Could you check a few things on this model? Use its own coordinates, in mm. A direction names the side the tool comes from. Round coordinates to 2 decimals unless told otherwise and drop trailing zeros. Loops run counter-clockwise (first coordinate to the right, second up) from the corner with the lowest first, then second, coordinate; pieces in that order, holes last. Notation, with made-up numbers: (-18.5, 39) -> (-2.5, 39) arc R11 cw to (-2.5, 53) -> close; hole circle Ø10 at (71.25, 40.25). An arc over 180 degrees is marked (long way). One line per item, written item: value.
```python
from build123d import *

# Parameters (mm, degrees)
F1_DEPTH = 20
F2_R     = 5
F4_R     = 2.5
F5_DEPTH = 62.5836819879


with BuildPart() as f1:
    # F0 (on Front) → F1 (new body, symmetric)
    with BuildSketch(Plane.XZ):
        with BuildLine():
            Line((37.7684786426, 214.1956862802), (38.6367195309, 219.1197250452))
            ThreePointArc((38.6367195309, 219.1197250452), (0, 222.5), (-38.6367195309, 219.1197250452))
            Line((-38.6367195309, 219.1197250452), (-37.7684786426, 214.1956862802))
            ThreePointArc((-37.7684786426, 214.1956862802), (-2.5001651855, 217.4856298104), (32.8344587783, 215.0073215422))
            ThreePointArc((32.8344587783, 215.0073215422), (35.3038012268, 214.6156835344), (37.7684786426, 214.1956862802))
        make_face()
        with BuildLine():
            Line((30.3884310917, 172.3413567771), (37.7684786426, 214.1956862802))
            ThreePointArc((37.7684786426, 214.1956862802), (35.3038012268, 214.6156835344), (32.8344587783, 215.0073215422))
            Line((32.8344587783, 215.0073215422), (25.451986353, 173.1392398929))
            ThreePointArc((25.451986353, 173.1392398929), (27.9230587413, 172.7579311943), (30.3884310917, 172.3413567771))
        make_face()
        with BuildLine():
            Line((29.5201902034, 167.4173180121), (30.3884310917, 172.3413567771))
            ThreePointArc((30.3884310917, 172.3413567771), (27.9230587413, 172.7579311943), (25.451986353, 173.1392398929))
            ThreePointArc((25.451986353, 173.1392398929), (-2.5002551932, 174.9821382998), (-30.3884310917, 172.3413567771))
            Line((-30.3884310917, 172.3413567771), (-29.5201902034, 167.4173180121))
            ThreePointArc((-29.5201902034, 167.4173180121), (0, 170), (29.5201902034, 167.4173180121))
        make_face()
    extrude(amount=F1_DEPTH, both=True)

    # F2
    f2_edges = [f1.edges().sort_by_distance(p)[0] for p in [
        (38.63672, 0, 219.119725),
        (32.834459, 0, 215.007322),
        (29.52019, 0, 167.417318),
        (25.451986, 0, 173.13924),
    ]]
    fillet(f2_edges, radius=F2_R)

    # F4 (on offset) → F5 (cut, through all)
    with BuildSketch(Plane.XY.offset(230)):
        with Locations((0, 12.5)):
            Circle(F4_R)
        with Locations((0, -12.5)):
            Circle(F4_R)
    extrude(amount=-F5_DEPTH, mode=Mode.SUBTRACT)


solid = f1.part
```
(1) Imagine slicing it at A-A on x = 0. Write out the boundary of the cut face in (y, z).
Results below:
outline: (-20, 170) -> (-15, 170) -> (-15, 175) -> (-20, 175) -> close; (-20, 217.5) -> (-15, 217.5) -> (-15, 222.5) -> (-20, 222.5) -> close; (-10, 170) -> (10, 170) -> (10, 175) -> (-10, 175) -> close; (-10, 217.5) -> (10, 217.5) -> (10, 222.5) -> (-10, 222.5) -> close; (15, 170) -> (20, 170) -> (20, 175) -> (15, 175) -> close; (15, 217.5) -> (20, 217.5) -> (20, 222.5) -> (15, 222.5) -> close
(2) Imagine slicing it at B-B on x = -15. Write out the boundary of the cut face in (y, z), then the cut area to 3 significant figures.
Results below:
outline: (-20, 169.34) -> (20, 169.34) -> (20, 174.36) -> (-20, 174.36) -> close; (-20, 216.98) -> (20, 216.98) -> (20, 221.99) -> (-20, 221.99) -> close
area: 401 mm²
(3) Imagine slicing it at D-D on y = 12.5. Give the number of separate pieces and of enclosed holes in the cut face, then the cut area to 3 significant figures.
Results below:
separate pieces: 3
enclosed holes: 0
area: 848 mm²
(4) Please list where these lines run through material, in increasing order: L1, parallel to Y at x = 0, z = 173; L2, parallel to Z at x = 0, y = 0; L3, parallel to Z at x = 4.5, y = 8.
Results below:
L1: y = -20 to -15, -10 to 10, 15 to 20
L2: z = 170 to 175, 217.5 to 222.5
L3: z = 169.94 to 174.94, 217.45 to 222.45
(5) On a 3-axis mill with a long thin cutter (end or side, diameter ignored), from which of +Z, -Z, +X, -X, +Y, -Y can I reach the whole of each face in a straight line? I mean faces 4 (the face through (5, 20, 218)), 5 (the face through (24.298, -0.28, 174.682)), 6 (the face through (29.15, -0.28, 194.11)). Say none if no direction works.
Results below:
face 4: +Z, -Z, +X, -X, +Y
face 5: +Y, -Y
face 6: -X, +Y, -Y
(6) We'd pull the mould along Z, two halves only. Please class faces 1 (the face through (-0.54, 10.06, 220.03)), 2 (the face through (-29.96, -0.28, 169.91)), 3 (the face through (-4.504, -0.28, 174.942)): +Z half, -Z half, draft (parallel to the pull), parting line (faces both ways), or undercut.
Results below:
face 1: draft
face 2: -Z half
face 3: undercut
(7) Imagine slicing it at C-C on x = -24.5. Write out the boundary of the cut face in (y, z), then the cut area to 3 significant figures.
Results below:
outline: (-20, 168.23) -> (20, 168.23) -> (20, 173.28) -> (-20, 173.28) -> close; (-20, 216.12) -> (20, 216.12) -> (20, 221.15) -> (-20, 221.15) -> close
area: 403 mm²
(8) For pin 1 Ø6 at (y, z) = (0, 195.5) entering from +X; pin 2 Ø6.5 at (x, y) = (0, -12.5) entering from -Z; pin 3 Ø5 at (y, z) = (14.5, 195) entering from -X; pin 4 Ø4 at (x, y) = (0, 12.5) entering from +Z, each with a flat end and sliding along its axis, tell me the tip position at first contact or that it passes through.
Results below:
pin 1: stops at x = 35
pin 2: stops at z = 169.97
pin 3: stops at x = 28.87
pin 4: passes through
